Verification items for this drawing (mm, ordinates from the low corner). Coordinates: 2 decimals unless noted, no trailing zeros. Write each loop counter-clockwise with the first axis right and the second up, starting at its lowest first coordinate (ties: lowest second). Pieces come first, ordered by that corner, then holes. Notation, with made-up numbers: M 43.25,49 L 58.25,49 A23 cw 58.25,64 Z; hole C 14.25,-1.75 d3. An arc over 180 degrees is marked long. Answer as CSV lines item,"result". Start each with the question number.
1) Section check B-B (x = 7). Record the cut outline in (y, z), and give its area (3 significant figures).
2) Go/stop test with flat-tipped pins: pin 1 Ø1.5 at (x, z) = (7.5, 111.5) entering from +Y; pin 2 Ø5 at (y, z) = (294.5, 85) entering from +X; pin 3 Ø1.5 at (x, z) = (8, 58.5) entering from -Y. Record where each tip stops, or that it passes through.
3) Material ranges on L1, parallel to Y at x = 5.5, z = 109, recorded low to high. Write a range as [from, to].
4) Section check A-A (z = 133.5). Record the cut outline in (x, y), and give its area (3 significant figures).
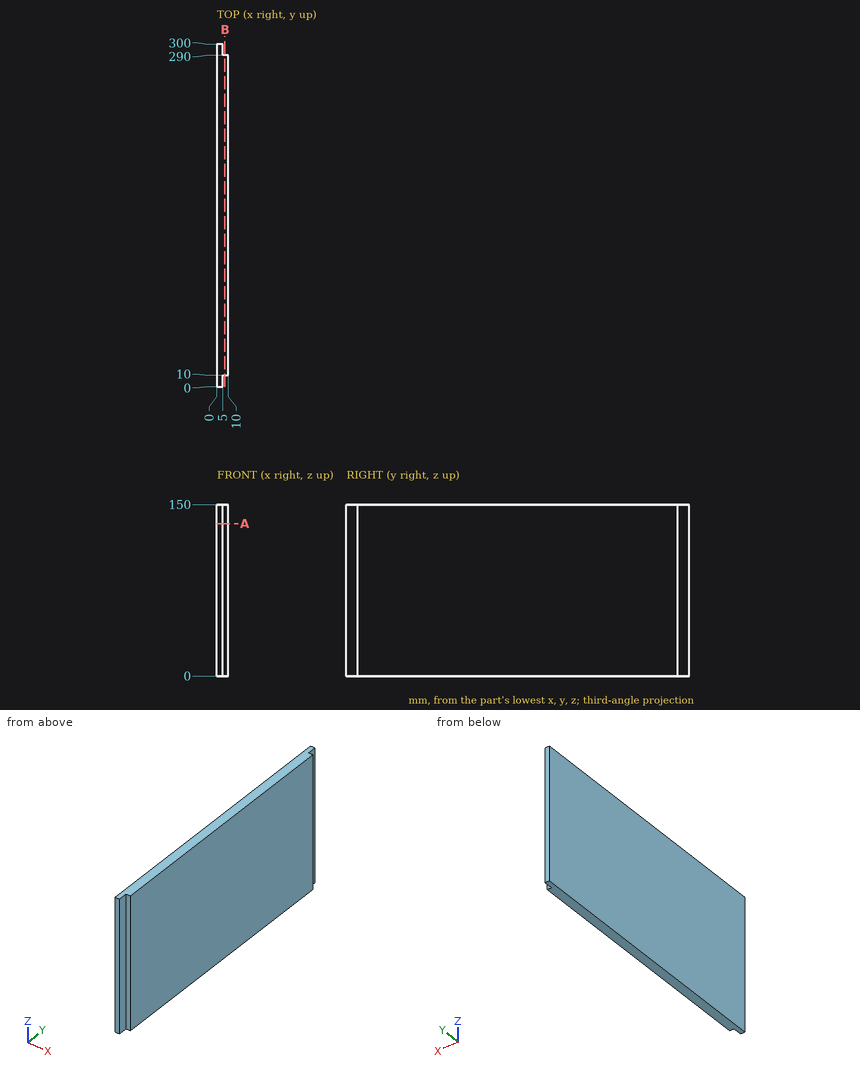
Results found:
1,outline,"M 10,0 L 290,0 L 290,150 L 10,150 Z"
1,area,"42,000 mm2"
2,pin 1,"stops at y = 290"
2,pin 2,"stops at x = 5"
2,pin 3,"stops at y = 10"
3,L1,"y = [10, 290]"
4,outline,"M 0,0 L 5,0 L 5,10 L 10,10 L 10,290 L 5,290 L 5,300 L 0,300 Z"
4,area,"2,900 mm2"
